Model file for the job. Use its own axes, mm. Round coordinates to 2 decimals unless told otherwise and drop trailing zeros. Order: outer loops, then holes, each group sorted by start corner. A loop starts at its lowest first (then second) coordinate and runs counter-clockwise, first axis right, second up. Notation, with made-up numbers: (0, 37.25) - (24, 37.25) arc R25 ccw to (24, 71.25) - close; hole circle Ø10 at (20, 15.5). An arc over 180 degrees is marked (long way). Answer as CSV lines item,"result". Start each with the question number.
1. Band-saw the part on D-D on x = -56. List the corners of the cut face in (y, z) (1 decimal), then the cut area to 3 significant figures.
2. Wall check: line 1 along X through (y, z) = (1.2, 0); line 2 along Z through (x, y) = (0, 1.7); line 3 along X through (y, z) = (2.4, -152.4). Give the ranges that are in metal, low to high. Write a range as [from, to].
3. Pull direction Z, two halves, no side cores. Call faces 1 (the face through (1, 0, -56)), 2 (the face through (-0.099, 1.565, -154.646)), 3 (the face through (-78.43, 1.57, -0.29)), 4 (the face through (-0.123, 1.565, -160.337)): released by +Z, released by -Z, zero draft, split by the parting line, or undercut.
4. Band-saw the part on A-A on y = 2.05. List the corners of the cut face in (x, z) (1 decimal).
5. Band-saw the part on B-B on z = 0. List the corners of the cut face in (x, y) (1 decimal), then the cut area to 3 significant figures.
6. Band-saw the part on C-C on z = -152.4. List the corners of the cut face in (x, y) (3 decimals), then the cut area to 3 significant figures.
7. Pin check, flat tips, straight feed: pin 1 Ø1 at (x, y) = (13, 2.5) entering from -Z; pin 2 Ø4 at (x, z) = (-76.2, 0) entering from +Y. Stop position of each tip, or through.
Autodesk Inventor part; units mm, degrees
ref_plane "YZ Plane" through (0, 0, 0) normal (1, 0, 0) x (0, 1, 0)
ref_plane "XZ Plane" through (0, 0, 0) normal (0, 1, 0) x (-1, 0, 0)
ref_plane "XY Plane" through (0, 0, 0) normal (0, 0, 1) x (1, 0, 0)
sketch "Sketch1" plane through (0, 0, 0) normal (0, 1, 0) x (-1, 0, 0)
  line L0 (76.2, 0) -> (-76.2, 0)
  line L1 (0, 0) -> (0, -152.4)
  line L2 (7.0995, -155.9498) -> (83.2995, -3.5498)
  line L3 (76.2, 7.9375) -> (-76.2, 7.9375)
  line L4 (-83.2995, -3.5498) -> (-7.0995, -155.9498)
  circle A0 centre (76.2, 0) radius 7.9375
  circle A1 centre (-76.2, 0) radius 7.9375
  circle A2 centre (0, -152.4) radius 7.9375
  dimension "d0" = 152.4
  dimension "d1" = 152.4
  dimension "d3" = 15.875
  dimension "d4" = 15.875
  dimension "d5" = 15.875
extrude "Extrusion1" add sketch "Sketch1" along normal blind 3.175
sketch "Sketch2" plane through (0, 3.175, 0) normal (0, 1, 0) x (1, 0, 0)
  arc A0 (-83.2995, 3.5498) -> (-76.2, -7.9375) centre (-76.2, 0) ccw
  line L0 (-76.2, -7.9375) -> (76.2, -7.9375)
  arc A1 (76.2, -7.9375) -> (83.2995, 3.5498) centre (76.2, 0) ccw
  line L1 (83.2995, 3.5498) -> (7.0995, 155.9498)
  arc A2 (7.0995, 155.9498) -> (-7.0995, 155.9498) centre (0, 152.4) ccw
  line L2 (-7.0995, 155.9498) -> (-83.2995, 3.5498)
  point P0 (0, 0)
hole "Hole1" at (-76.2, 3.175, 0) at (76.2, 3.175, 0) at (0, 3.175, -152.4) direction (0, -1, 0) diameter 4.4958 end through all
properties part number "Bed Support"
Reply:
1,outline,"(0, -58.1) - (3.2, -58.1) - (3.2, 7.9) - (0, 7.9) - close"
1,area,"210 mm2"
2,line 1,"x = [-84.14, -78.45], [-73.95, 73.95], [78.45, 84.14]"
2,line 2,"z = [-160.34, -154.65], [-150.15, 7.94]"
2,line 3,"x = [-8.87, -2.25], [2.25, 8.87]"
3,face 1,"zero draft"
3,face 2,"undercut"
3,face 3,"undercut"
3,face 4,"released by -Z"
4,outline,"(-83.3, -3.5) - (-7.1, -155.9) arc R7.9 ccw to (7.1, -155.9) - (83.3, -3.5) arc R7.9 ccw to (76.2, 7.9) - (-76.2, 7.9) arc R7.9 ccw to start; hole circle Ø4.5 at (-76.2, 0); hole circle Ø4.5 at (0, -152.4); hole circle Ø4.5 at (76.2, 0)"
5,outline,"(-84.1, 0) - (-78.4, 0) - (-78.4, 3.2) - (-84.1, 3.2) - close; (-74, 0) - (74, 0) - (74, 3.2) - (-74, 3.2) - close; (78.4, 0) - (84.1, 0) - (84.1, 3.2) - (78.4, 3.2) - close"
5,area,"506 mm2"
6,outline,"(-8.874, 0) - (-2.248, 0) - (-2.248, 3.175) - (-8.874, 3.175) - close; (2.248, 0) - (8.874, 0) - (8.874, 3.175) - (2.248, 3.175) - close"
6,area,"42.1 mm2"
7,pin 1,"stops at z = -145.15"
7,pin 2,"passes through"
